For this review, take the finished solid that the model builds, in its own axes (mm). Face numbers are marked on the shaded views. A direction names the side the tool comes from. Round coordinates to 2 decimals unless told otherwise and drop trailing zeros. Order: outer loops, then holes, each group sorted by start corner. A loop starts at its lowest first (then second) coordinate and runs counter-clockwise, first axis right, second up.
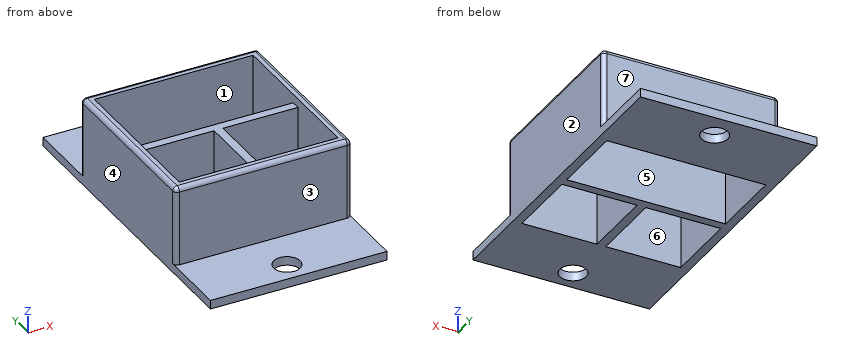
```python
from build123d import *

# Parameters (mm, degrees)
F0_W     = 20
F0_H     = 20
F1_DEPTH = 10
F2_T     = -1
F4_DEPTH = 9
F5_W     = 20
F5_H     = 8
F5_R     = 1.5
F6_DEPTH = 1
F7_W     = 18
F7_H     = 18
F8_DEPTH = 1
F9_R     = 0.5


with BuildPart() as f1:
    # F0 (on Top) → F1 (new body)
    with BuildSketch(Plane.XY):
        Rectangle(F0_W, F0_H)
    extrude(amount=F1_DEPTH)

    # F2
    f2_openings = [f1.faces().sort_by_distance(p)[0] for p in [
        (0, 0, 0),
    ]]
    offset(amount=F2_T, openings=f2_openings)

    # F3 (on Top) → F4 (join)
    with BuildSketch(Plane.XY):
        Polygon((-0.5, -9), (0.5, -9), (0.5, -0.5), (9, -0.5), (9, 0.5), (0.5, 0.5), (-0.5, 0.5), (-9, 0.5), (-9, -0.5), (-0.5, -0.5), align=None)
    extrude(amount=F4_DEPTH)

    # F5 (on Top) → F6 (join)
    with BuildSketch(Plane.XY):
        with Locations((0, -13.5)):
            Rectangle(F5_W, F5_H)
        with Locations((0, -15)):
            Circle(F5_R, mode=Mode.SUBTRACT)
        with Locations((0, 14)):
            Rectangle(F5_W, F5_H)
        with Locations((0, 15)):
            Circle(F5_R, mode=Mode.SUBTRACT)
    extrude(amount=F6_DEPTH)

    # F7 (on face) → F8 (cut)
    with BuildSketch(Plane.XY.offset(10)):
        Rectangle(F7_W, F7_H)
    extrude(amount=-F8_DEPTH, mode=Mode.SUBTRACT)

    # F9
    f9_edges = [f1.edges().sort_by_distance(p)[0] for p in [
        (10, 0, 10),
        (0, -10, 10),
        (10, -10, 5.5),
        (-10, -10, 5.5),
        (10, 10, 5.5),
        (-10, 10, 5.5),
        (0, 10, 10),
        (-10, 0, 10),
    ]]
    fillet(f9_edges, radius=F9_R)


solid = f1.part
```
Q1. Take a section at C-C, the plane y = 15. State the section outline as (x, z) points.
Q2. Wall thickness on line 1 (Y direction, x = 0, z = 0.2); line 2 (X direction, y = -6.5, z = 6.25): over which ranges is each line inside the solid? List them lowest first.
Q3. Take a section at D-D, the plane x = -6. State the section outline as (y, z) points, plus the area to 3 significant figures.
Q4. Take a section at B-B, the plane z = 7.25. State the section outline as (x, y) points.
Q5. Take a section at A-A, the plane x = 0. State the section outline as (y, z) points, plus the area to 3 significant figures.
Q6. Tool access review of the marked faces 1, 2 and 3: name each direction out of +Z, -Z, +X, -X, +Y, -Y from which nothing blocks a thin tool from reaching the whole face with its end or side.
Q7. Mouldability with a two-part tool opening along Y and no side actions: class the marked faces 4, 5, 6 and 7 as +Y half, -Y half, draft (parallel to the pull), parting line (faces both ways), or undercut.
Q8. Clearance check with flat-ended pins moving along their axes: pin 1 (4 mm diameter, centred on x = 0, y = -15, fed in from +Z); pin 2 (2.5 mm diameter, centred on x = 6.5, z = 3, fed in from -Y); pin 3 (2.5 mm diameter, centred on x = -2, z = 6, fed in from +Y). State where each tip first meets the part, or that it passes through.
Working result:
1. outline: (-10, 0) - (-1.5, 0) - (-1.5, 1) - (-10, 1) - close; (1.5, 0) - (10, 0) - (10, 1) - (1.5, 1) - close
2. line 1: y = -17.5 to -16.5, -13.5 to 0.5, 9 to 13.5, 16.5 to 18
2. line 2: x = -10 to -9, -0.5 to 0.5, 9 to 10
3. outline: (-17.5, 0) - (-9, 0) - (-9, 10) - (-9.5, 10) arc R0.5 ccw to (-10, 9.5) - (-10, 1) - (-17.5, 1) - close; (-0.5, 0) - (0.5, 0) - (0.5, 9) - (-0.5, 9) - close; (9, 0) - (18, 0) - (18, 1) - (10, 1) - (10, 9.5) arc R0.5 ccw to (9.5, 10) - (9, 10) - close
3. area: 44.4 mm2
4. outline: (-10, -9.5) arc R0.5 ccw to (-9.5, -10) - (9.5, -10) arc R0.5 ccw to (10, -9.5) - (10, 9.5) arc R0.5 ccw to (9.5, 10) - (-9.5, 10) arc R0.5 ccw to (-10, 9.5) - close; hole (-9, -9) - (-0.5, -9) - (-0.5, -0.5) - (-9, -0.5) - close; hole (-9, 0.5) - (9, 0.5) - (9, 9) - (-9, 9) - close; hole (0.5, -9) - (9, -9) - (9, -0.5) - (0.5, -0.5) - close
5. outline: (-17.5, 0) - (-16.5, 0) - (-16.5, 1) - (-17.5, 1) - close; (-13.5, 0) - (0.5, 0) - (0.5, 9) - (-9, 9) - (-9, 10) - (-9.5, 10) arc R0.5 ccw to (-10, 9.5) - (-10, 1) - (-13.5, 1) - close; (9, 0) - (13.5, 0) - (13.5, 1) - (10, 1) - (10, 9.5) arc R0.5 ccw to (9.5, 10) - (9, 10) - close; (16.5, 0) - (18, 0) - (18, 1) - (16.5, 1) - close
5. area: 115 mm2
6. face 1: +Z, -Z
6. face 2: +Z, -Z, +X, +Y, -Y
6. face 3: +Z, +X, -X, -Y
7. face 4: draft
7. face 5: undercut
7. face 6: undercut
7. face 7: +Y half
8. pin 1: stops at z = 1
8. pin 2: stops at y = -10
8. pin 3: stops at y = 10
